Part print with two shaded views. Sizes in mm from the minimum x, y, z corner. A direction names the side the tool comes from. Coordinates: 2 decimals unless noted, no trailing zeros. Order: outer loops, then holes, each group sorted by start corner. A loop starts at its lowest first (then second) coordinate and runs counter-clockwise, first axis right, second up. Notation, with made-up numbers: M 31,63.25 L 72,63.25 A18 cw 72,83.25 Z; hole C 88,57 d2. An arc over 180 degrees is marked long. Answer in a Markdown table with one row per item. Add a question column.
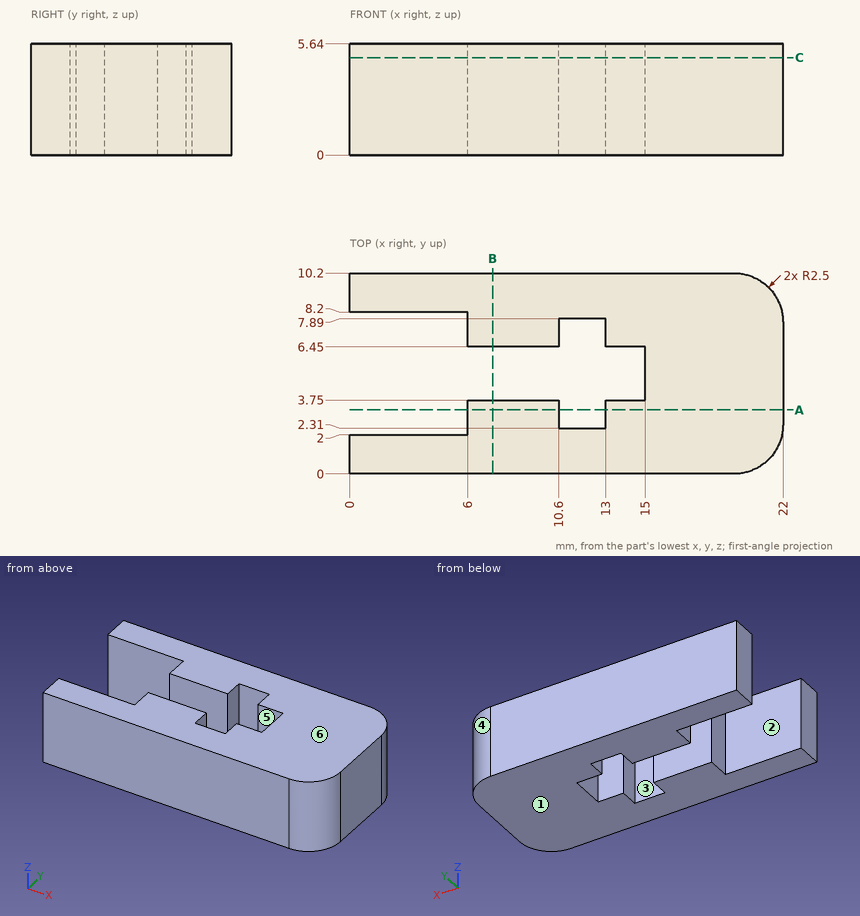
(1) Slice it at C-C (z = 4.95). List the corners of the cut face in (x, y), and give its area (3 significant figures).
(2) Pull direction Y, two halves, no side cores. Call the marked faces 4, 5 and 6: pulls with the +Y half, pulls with the -Y half, needs draft (parallel to the pull), parting line crosses it, or undercut.
(3) Wall check: line 1 (X direction, y = 7.5, z = 3.75); line 2 (Y direction, x = 11.25, z = 0.5); line 3 (Y direction, x = 7.75, z = 3). Give the ranges that are in metal, low to high.
(4) Slice it at B-B (x = 7.25). List the corners of the cut face in (y, z).
(5) Slice it at A-A (y = 3.25). List the corners of the cut face in (x, z).
(6) Drop flat-ended pins along their axis: P1, Ø2, axis at y = 5.5, z = 3.5, coming from the -X side; P2, Ø1.5, axis at x = 11.5, y = 3, coming from the -Z side. Give the stop position or say it passes through.
(7) 3-axis set-ups, long thin cutter, end or side, ignore diameter. For the marked faces 1, 2 and 3: which of +Z, -Z, +X, -X, +Y, -Y reach the whole face in a straight line?
Computed:
| question | item | result |
|---|---|---|
| 1 | outline | M 0,0 L 19.5,0 A2.5 ccw 22,2.5 L 22,7.7 A2.5 ccw 19.5,10.2 L 0,10.2 L 0,8.2 L 6,8.2 L 6,6.45 L 10.6,6.45 L 10.6,7.89 L 13,7.89 L 13,6.45 L 15,6.45 L 15,3.75 L 13,3.75 L 13,2.31 L 10.6,2.31 L 10.6,3.75 L 6,3.75 L 6,2 L 0,2 Z |
| 1 | area | 153 mm^2 |
| 2 | face 4 | pulls with the +Y half |
| 2 | face 5 | undercut |
| 2 | face 6 | needs draft |
| 3 | line 1 | x = 6 to 10.6, 13 to 22 |
| 3 | line 2 | y = 0 to 2.31, 7.89 to 10.2 |
| 3 | line 3 | y = 0 to 3.75, 6.45 to 10.2 |
| 4 | outline | M 0,0 L 3.75,0 L 3.75,5.64 L 0,5.64 Z; M 6.45,0 L 10.2,0 L 10.2,5.64 L 6.45,5.64 Z |
| 5 | outline | M 6,0 L 10.6,0 L 10.6,5.64 L 6,5.64 Z; M 13,0 L 22,0 L 22,5.64 L 13,5.64 Z |
| 6 | P1 | stops at x = 6 |
| 6 | P2 | stops at z = 0 |
| 7 | face 1 | -Z, +X, -X, +Y, -Y |
| 7 | face 2 | +Z, -Z, -X |
| 7 | face 3 | +Z, -Z |
